Input: dimensioned drawing with shaded views. Units: mm. Origin: part minimum x, y, z. Round coordinates to 2 decimals unless told otherwise and drop trailing zeros. Write each loop counter-clockwise with the first axis right and the second up, starting at its lowest first coordinate (ties: lowest second). Pieces come first, ordered by that corner, then holes. Notation, with made-up numbers: (-40, 7.5) -> (15, 7.5) arc R18 ccw to (15, 29.5) -> close; hole circle Ø7 at (6, 73.5). An arc over 180 degrees is marked (long way). Use one line per item in the form item = value. Start each with the question number.
1. Cut plane D-D, the plane x = 4. Return the cut outline in (y, z) (1 decimal).
2. Cut plane B-B, the plane z = 0.3. Return the cut outline in (x, y) (1 decimal), plus the area to 3 significant figures.
3. Line query: L1, parallel to X at y = 8.25, z = 0.4 (1 decimal); L2, parallel to X at y = 10.25, z = 0.5 (1 decimal); L3, parallel to Y at x = 19, z = 0.7. Output: solid intervals per line, ascending.
4. Cut plane C-C, the plane y = 9.5. Return the cut outline in (x, z) (1 decimal).
5. Cut plane A-A, the plane x = 20.5. Return the cut outline in (y, z).
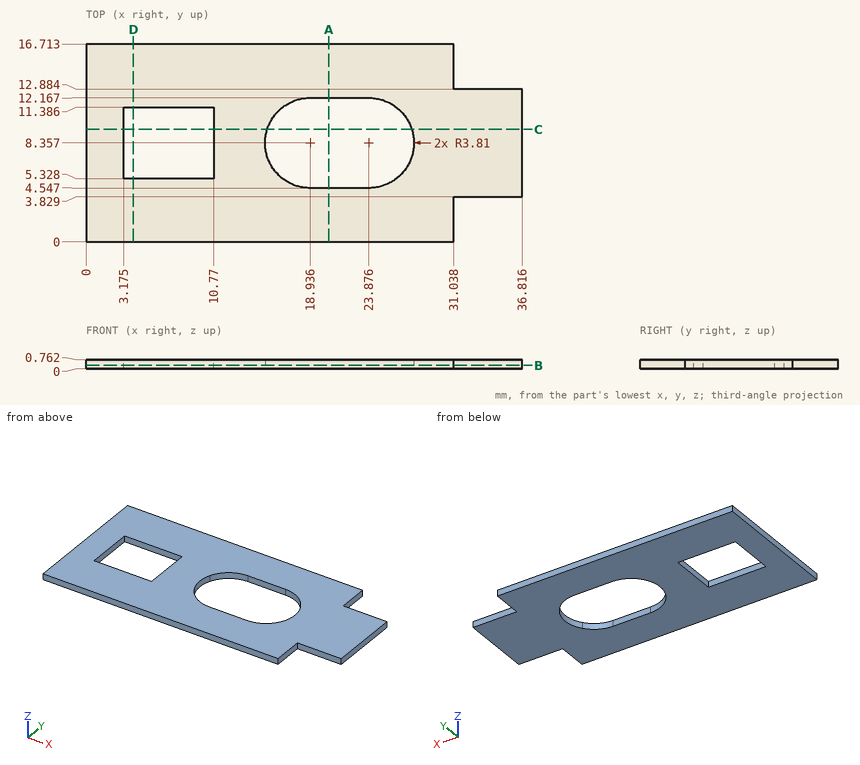
Outcome:
q1.outline = (0, 0) -> (5.3, 0) -> (5.3, 0.8) -> (0, 0.8) -> close; (11.4, 0) -> (16.7, 0) -> (16.7, 0.8) -> (11.4, 0.8) -> close
q2.outline = (0, 0) -> (31, 0) -> (31, 3.8) -> (36.8, 3.8) -> (36.8, 12.9) -> (31, 12.9) -> (31, 16.7) -> (0, 16.7) -> close; hole (3.2, 5.3) -> (10.8, 5.3) -> (10.8, 11.4) -> (3.2, 11.4) -> close; hole (18.9, 4.5) -> (23.9, 4.5) arc R3.8 ccw to (23.9, 12.2) -> (18.9, 12.2) arc R3.8 ccw to start
q2.area = 442 mm^2
q3.L1 = 0 to 3.2, 10.8 to 15.1, 27.7 to 36.8
q3.L2 = 0 to 3.2, 10.8 to 15.6, 27.2 to 36.8
q3.L3 = 0 to 4.55, 12.17 to 16.71
q4.outline = (0, 0) -> (3.2, 0) -> (3.2, 0.8) -> (0, 0.8) -> close; (10.8, 0) -> (15.3, 0) -> (15.3, 0.8) -> (10.8, 0.8) -> close; (27.5, 0) -> (36.8, 0) -> (36.8, 0.8) -> (27.5, 0.8) -> close
q5.outline = (0, 0) -> (4.55, 0) -> (4.55, 0.76) -> (0, 0.76) -> close; (12.17, 0) -> (16.71, 0) -> (16.71, 0.76) -> (12.17, 0.76) -> close
